CAD build for the part. Positions are in the model's coordinates, mm. Coordinates: 2 decimals unless noted, no trailing zeros. Loops run counter-clockwise (first coordinate to the right, second up) from the corner with the lowest first, then second, coordinate; pieces in that order, holes last. Notation, with made-up numbers: (-5, 0.25) -> (8, 0.25) arc R25 cw to (8, 14.25) -> close; hole circle Ø8 at (78.25, -29.5). An arc over 180 degrees is marked (long way). Write each question's results on one line, items separated by ' | '.
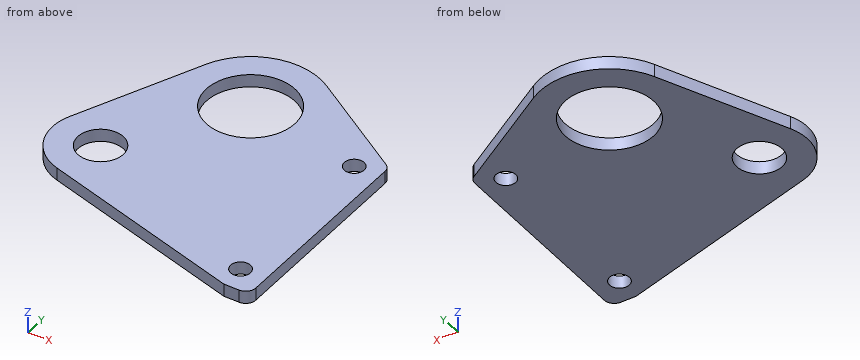
```python
from build123d import *

# Parameters (mm, degrees)
SKETCH1_W                  = 76.2
SKETCH1_H                  = 76.2
BOSS_EXTRUDE1_DEPTH        = 3.175
F_9_0_196_DIAMETER_HOLE1_D = 4.9784
SKETCH4_R                  = 5.715
SKETCH4_R_2                = 11.1125
CUT_EXTRUDE1_DEPTH         = 3.175
CUT_EXTRUDE2_DEPTH         = 3.175
FILLET1_R                  = 2.54


with BuildPart() as part:
    # Sketch1 → Boss-Extrude1 (new body)
    with BuildSketch(Plane(origin=(0, 0, 0), x_dir=(0, 1, 0), z_dir=(0, 0, 1))):
        Rectangle(SKETCH1_W, SKETCH1_H)
    extrude(amount=BOSS_EXTRUDE1_DEPTH)

    # #9 (0.196) Diameter Hole1 (through all)
    with Locations(Plane.XY.offset(3.175)):
        with Locations((31.75, -31.75), (31.75, 11.43)):
            Hole(F_9_0_196_DIAMETER_HOLE1_D / 2)

    # Sketch4 → Cut-Extrude1 (cut)
    with BuildSketch(Plane.XY.offset(3.175)):
        with Locations((-16.587404081, -11.717617647)):
            Circle(SKETCH4_R)
        with Locations((2.053516604, 17.062934398)):
            Circle(SKETCH4_R_2)
    extrude(amount=-CUT_EXTRUDE1_DEPTH, mode=Mode.SUBTRACT)

    # Sketch6 → Cut-Extrude2 (cut)
    with BuildSketch(Plane.XY.offset(3.175)):
        with BuildLine():
            Line((11.387489681, 31.821520131), (38.1, 14.927363968))
            Line((38.1, 14.927363968), (38.1, 38.1))
            Line((38.1, 38.1), (-38.1, 38.1))
            Line((-38.1, 38.1), (-38.1, -38.1))
            Line((-38.1, -38.1), (31.75, -38.1))
            Line((31.75, -38.1), (-19.906877313, -23.316984977))
            ThreePointArc((-19.906877313, -23.316984977), (-27.515067303, -16.831363975), (-27.620065644, -6.834523972))
            Line((-27.620065644, -6.834523972), (-13.914809342, 24.13056998))
            ThreePointArc((-13.914809342, 24.13056998), (-3.025000705, 33.770644241), (11.387489681, 31.821520131))
        make_face()
    extrude(amount=-CUT_EXTRUDE2_DEPTH, mode=Mode.SUBTRACT)

    # Fillet1
    fillet1_edges = [part.edges().sort_by_distance(p)[0] for p in [
        (38.1, 14.927363968, 1.5875),
        (38.1, -38.1, 1.5875),
    ]]
    fillet(fillet1_edges, radius=FILLET1_R)


solid = part.part
```
Q1. Cut at A-A on y = 21. Write the cut outline in (x, z) (3 decimals), and give its area (3 significant figures).
Results are:
outline: (-15.3, 0) -> (-8.338, 0) -> (-8.338, 3.175) -> (-15.3, 3.175) -> close; (12.445, 0) -> (28.498, 0) -> (28.498, 3.175) -> (12.445, 3.175) -> close | area: 73.1 mm^2
Q2. Cut at D-D on x = -23.5. Write the cut outline in (y, z) (3 decimals), and give its area (3 significant figures).
Results are:
outline: (-21.606, 0) -> (2.474, 0) -> (2.474, 3.175) -> (-21.606, 3.175) -> close | area: 76.5 mm^2
Q3. Cut at B-B on x = -2. Write the cut outline in (y, z) (3 decimals).
Results are:
outline: (-28.442, 0) -> (6.716, 0) -> (6.716, 3.175) -> (-28.442, 3.175) -> close; (27.41, 0) -> (34.048, 0) -> (34.048, 3.175) -> (27.41, 3.175) -> close
Q4. Cut at C-C on y = -3.5. Write the cut outline in (x, z) (3 decimals), and give its area (3 significant figures).
Results are:
outline: (-26.144, 0) -> (38.1, 0) -> (38.1, 3.175) -> (-26.144, 3.175) -> close | area: 204 mm^2
Q5. Wall check: L1, parallel to Y at x = 31.75, z = 1.15; L2, parallel to X at y = -11.5, z = 2.6; L3, parallel to Y at x = -13.5, z = 2.5. Give the ranges that are in metal, low to high. Write a range as from..to.
Results are:
L1: -38.1..-34.24, -29.26..8.94, 13.92..18.94 | L2: -28.65..-22.3, -10.88..38.1 | L3: -25.15..-16.53, -6.91..25
Q6. Drop flat-ended pins along their axis: pin 1 (1.5 mm diameter, centred on x = -5, z = 1, fed in from -Y); pin 2 (1.5 mm diameter, centred on x = 20, z = 1.5, fed in from -Y); pin 3 (1 mm diameter, centred on x = -18, z = 0.5, fed in from +Y). Give the stop position or say it passes through.
Results are:
pin 1: y = -27.8 | pin 2: y = -34.95 | pin 3: y = 16.03
